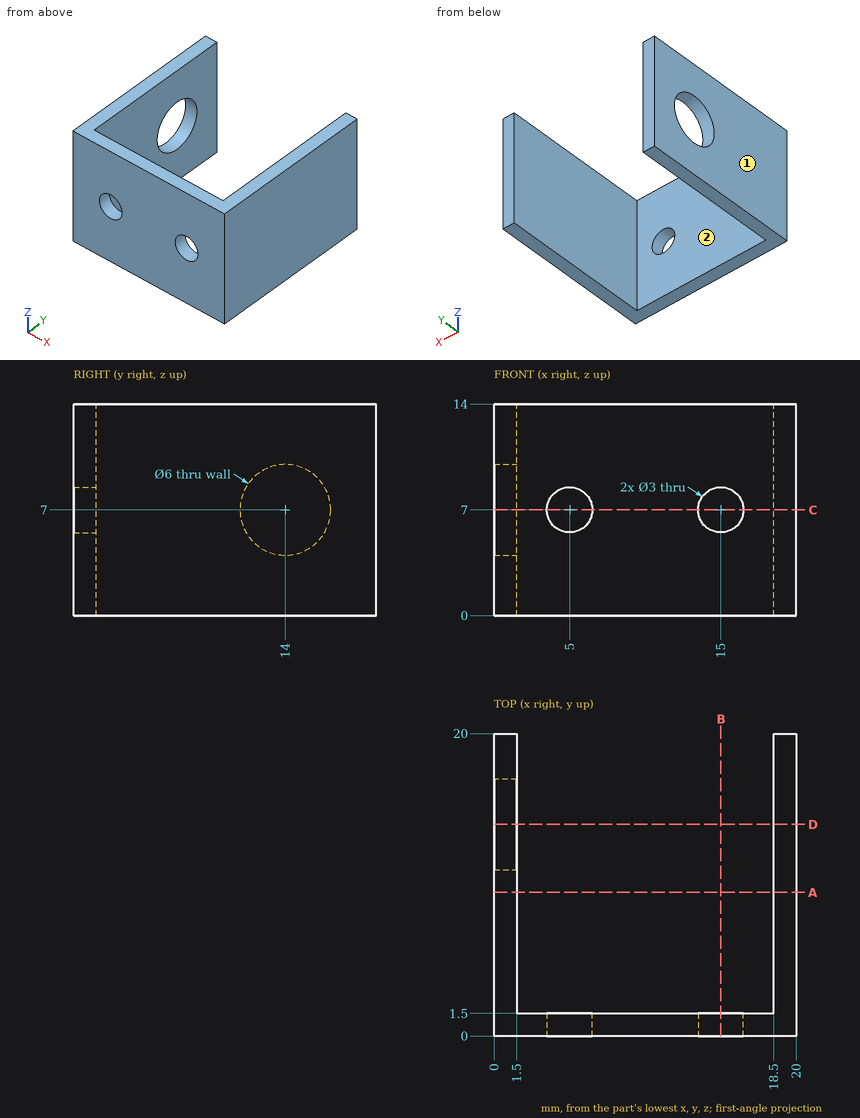
Can you work these out from the drawing? Everything is in mm from the part's minimum corner. A direction names the side the tool comes from. Round coordinates to 2 decimals unless told otherwise and drop trailing zeros. Write each loop counter-clockwise with the first axis right and the second up, starting at its lowest first coordinate (ties: lowest second). Pieces come first, ordered by that corner, then holes.
1. Suppose I cut it at C-C (z = 7). List the corners of the cut face in (x, y) for me, and give its area (3 significant figures).
2. Suppose I cut it at D-D (y = 14). List the corners of the cut face in (x, z) for me, and give its area (3 significant figures).
3. Suppose I cut it at B-B (x = 15). List the corners of the cut face in (y, z) for me.
4. I need wall thicknesses on L1, parallel to X at y = 9.5, z = 4; L2, parallel to Z at x = 5, y = 0.8; L3, parallel to Z at x = 1.15, y = 14. Which ranges of each line are inside material? Lowest first, please.
5. Will this pin go through, and if not, where does the flat tip stop? pin 1 Ø5 at (x, z) = (5, 7) entering from +Y.
6. Suppose I cut it at A-A (y = 9.5). List the corners of the cut face in (x, z) for me.
7. For the marked faces 1 and 2, which set-ups out of +Z, -Z, +X, -X, +Y, -Y let a thin tool reach every point of the face, with its end or its side?
Answer sheet:
1. outline: (0, 0) - (3.5, 0) - (3.5, 1.5) - (1.5, 1.5) - (1.5, 11) - (0, 11) - close; (0, 17) - (1.5, 17) - (1.5, 20) - (0, 20) - close; (6.5, 0) - (13.5, 0) - (13.5, 1.5) - (6.5, 1.5) - close; (16.5, 0) - (20, 0) - (20, 20) - (18.5, 20) - (18.5, 1.5) - (16.5, 1.5) - close
1. area: 67.5 mm2
2. outline: (0, 0) - (1.5, 0) - (1.5, 4) - (0, 4) - close; (0, 10) - (1.5, 10) - (1.5, 14) - (0, 14) - close; (18.5, 0) - (20, 0) - (20, 14) - (18.5, 14) - close
2. area: 33.0 mm2
3. outline: (0, 0) - (1.5, 0) - (1.5, 5.5) - (0, 5.5) - close; (0, 8.5) - (1.5, 8.5) - (1.5, 14) - (0, 14) - close
4. L1: x = 0 to 1.5, 18.5 to 20
4. L2: z = 0 to 5.5, 8.5 to 14
4. L3: z = 0 to 4, 10 to 14
5. pin 1: stops at y = 1.5
6. outline: (0, 0) - (1.5, 0) - (1.5, 14) - (0, 14) - close; (18.5, 0) - (20, 0) - (20, 14) - (18.5, 14) - close
7. face 1: +Z, -Z, -X, +Y, -Y
7. face 2: +Z, -Z, +Y
